Part model, mm, in its own coordinate system. A direction names the side the tool comes from. Round coordinates to 2 decimals unless told otherwise and drop trailing zeros. Order: outer loops, then holes, each group sorted by start corner. A loop starts at its lowest first (then second) coordinate and runs counter-clockwise, first axis right, second up. Notation, with made-up numbers: M -3.5,67 L 3.5,67 A19 cw 3.5,94 Z; hole C -24,-1 d9. An arc over 180 degrees is marked long. Write each question's results on one line, items separated by ' | '. Start each with the question number.
1. Band-saw the part on A-A, the plane y = 12. List the corners of the cut face in (x, z), then the cut area to 3 significant figures.
2. Band-saw the part on D-D, the plane y = -6. List the corners of the cut face in (x, z).
3. Which spindle directions (+Z, -Z, +X, -X, +Y, -Y) get a long thin tool onto all of the face, cutting with end or side? Do faces 5 (the face through (9, -6, -2.5)), 6 (the face through (-7.785, -14.465, -0.035)), 7 (the face through (9.25, 10, 5)). Say none if no direction does.
4. Band-saw the part on B-B, the plane z = -7.5. List the corners of the cut face in (x, y), then the cut area to 3 significant figures.
5. Drop flat-ended pins along their axis: pin 1 Ø4 at (x, z) = (-12.5, 1.5) entering from -Y; pin 2 Ø17.5 at (x, y) = (3.5, -4.5) entering from -Z; pin 3 Ø7 at (y, z) = (-2.5, -1.5) entering from -X. Give the stop position or say it passes through.
6. Probe L1, parallel to Y at x = 14, z = 7.5; L2, parallel to Z at x = -3.5, y = 9.5; L3, parallel to Y at x = -8.5, z = -7.5. List the from-to ranges inside material, lowest first. Write a range as [from, to].
7. Two-plate mould, pull along Y, no slides. Class faces 1 (the face through (3, -17, 0)), 2 (the face through (9.25, 10, -10)), 3 (the face through (-10.25, -3, 0)), 4 (the face through (0, 17, 0)): +Y half, -Y half, draft (parallel to the pull), parting line (faces both ways), or undercut.
8. Band-saw the part on C-C, the plane x = -2. List the corners of the cut face in (y, z).
```python
from build123d import *

# Parameters (mm, degrees)
SKETCH_1_W                  = 30
SKETCH_1_H                  = 34
EXTRUDE_1_DEPTH             = 16.25
SKETCH_2_W                  = 12.5
SKETCH_2_H                  = 24
CUT_EXTRUDE_1_DEPTH         = 40.626380102
SKETCH_5_W                  = 6
SKETCH_5_H                  = 24
CUT_EXTRUDE_2_DEPTH         = 49.521258228
HOLE_WIZARD_1_D             = 14
HOLE_WIZARD_1_2_D           = 5.5
HOLE_WIZARD_1_2_CBORE_D     = 9.4
HOLE_WIZARD_1_2_CBORE_DEPTH = 7
FILLET_1_R                  = 2
CHAMFER_1_SIZE              = 5


with BuildPart() as part:
    # 草图1 → 凸台-拉伸1 (new, symmetric)
    with BuildSketch(Plane(origin=(0, 0, 0), x_dir=(0, 0, -1), z_dir=(1, 0, 0))):
        Rectangle(SKETCH_1_W, SKETCH_1_H)
    extrude(amount=EXTRUDE_1_DEPTH, both=True)

    # 草图2 → 切除-拉伸1 (cut, through all)
    with BuildSketch(Plane(origin=(16.25, 0, 0), x_dir=(0, 0, -1), z_dir=(1, 0, 0))):
        with Locations((8.75, -5)):
            Rectangle(SKETCH_2_W, SKETCH_2_H)
        with Locations((-8.75, -5)):
            Rectangle(SKETCH_2_W, SKETCH_2_H)
    extrude(amount=-CUT_EXTRUDE_1_DEPTH, mode=Mode.SUBTRACT)

    # 草图5 → 切除-拉伸2 (cut, through all)
    with BuildSketch(Plane(origin=(0, 17.5, -15), x_dir=(1, 0, 0), z_dir=(0, 0, 1))):
        with Locations((-13.25, -22.5)):
            Rectangle(SKETCH_5_W, SKETCH_5_H)
    extrude(amount=CUT_EXTRUDE_2_DEPTH, mode=Mode.SUBTRACT)

    # Hole Wizard 1 (through all)
    with Locations(Plane.XY.offset(15)):
        with Locations((1.75, -6)):
            Hole(HOLE_WIZARD_1_D / 2)

    # Hole Wizard 1 2 (through all)
    with Locations(Plane(origin=(16.25, 0, 0), x_dir=(0, 0, -1), z_dir=(1, 0, 0))):
        with Locations((7.5, 12), (-7.5, 12)):
            CounterBoreHole(HOLE_WIZARD_1_2_D / 2, HOLE_WIZARD_1_2_CBORE_D / 2, HOLE_WIZARD_1_2_CBORE_DEPTH)

    # 圆角1
    fillet_1_edges = [part.edges().sort_by_distance(p)[0] for p in [
        (3, 7, 2.5),
        (3, 7, -2.5),
    ]]
    fillet(fillet_1_edges, radius=FILLET_1_R)

    # 倒角1
    chamfer_1_edges = [part.edges().sort_by_distance(p)[0] for p in [
        (16.25, -17, 0),
        (-10.25, -17, 0),
    ]]
    chamfer(chamfer_1_edges, length=CHAMFER_1_SIZE)


solid = part.part
```
Solution:
1) outline: M -16.25,-15 L 16.25,-15 L 16.25,-12.2 L 9.25,-12.2 L 9.25,-10.25 L -16.25,-10.25 Z; M -16.25,-4.75 L 9.25,-4.75 L 9.25,-2.8 L 16.25,-2.8 L 16.25,2.8 L 9.25,2.8 L 9.25,4.75 L -16.25,4.75 Z; M -16.25,10.25 L 9.25,10.25 L 9.25,12.2 L 16.25,12.2 L 16.25,15 L -16.25,15 Z | area: 563 mm^2
2) outline: M -10.25,-2.5 L -5.25,-2.5 L -5.25,2.5 L -10.25,2.5 Z; M 8.75,-2.5 L 16.25,-2.5 L 16.25,2.5 L 8.75,2.5 Z
3) face 5: -Z, +X, -X, -Y | face 6: +Z, -Z, -X, -Y | face 7: +X
4) outline: M -16.25,7 L 16.25,7 L 16.25,7.3 L 9.25,7.3 L 9.25,9.25 L -16.25,9.25 Z; M -16.25,14.75 L 9.25,14.75 L 9.25,16.7 L 16.25,16.7 L 16.25,17 L -16.25,17 Z | area: 119 mm^2
5) pin 1: y = 7 | pin 2: z = -2.5 | pin 3: x = -10.25
6) L1: [7, 7.3], [16.7, 17] | L2: [-15, -8.65], [-6.35, 6.35], [8.65, 15] | L3: [7, 9.25], [14.75, 17]
7) face 1: -Y half | face 2: undercut | face 3: draft | face 4: +Y half
8) outline: M -17,-2.5 L -11.91,-2.5 L -11.91,2.5 L -17,2.5 Z; M -0.09,-2.5 L 5,-2.5 A2 cw 7,-4.5 L 7,-15 L 17,-15 L 17,15 L 7,15 L 7,4.5 A2 cw 5,2.5 L -0.09,2.5 Z; hole C 12,-7.5 d5.5; hole C 12,7.5 d5.5
